Here's the drawing with two shaded views (mm, measured from the low corner). I have some questions. A direction names the side the tool comes from. Give positions to 0.01 mm unless a question says otherwise; leave off trailing zeros. Order: outer loops, then holes, each group sorted by start corner. A loop starts at its lowest first (then second) coordinate and runs counter-clockwise, first axis right, second up. Notation, with made-up numbers: M -21.75,50.25 L 30.25,50.25 A27 ccw 30.25,80.25 Z; hole C 63.25,-13.75 d11. An arc over 180 degrees is marked long. Write each question's results on one line, items separated by ' | '.
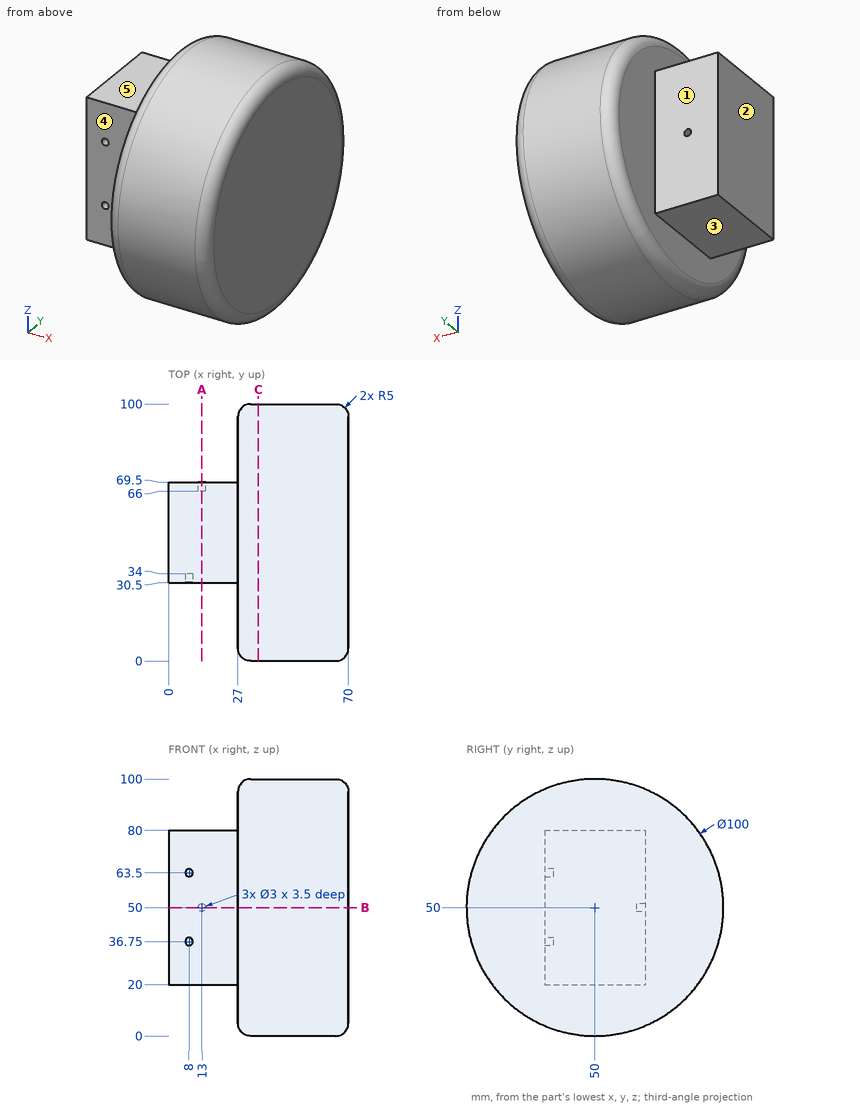
(1) For the marked faces 1, 2, 3, 4 and 5, which set-ups out of +Z, -Z, +X, -X, +Y, -Y let a thin tool reach every point of the face, with its end or its side?
Data:
face 1: +Z, -Z, -X, +Y | face 2: +Z, -Z, -X, +Y, -Y | face 3: -Z, -X, +Y, -Y | face 4: +Z, -Z, -X, -Y | face 5: +Z, -X, +Y, -Y
(2) I need wall thicknesses on L1, parallel to X at y = 68, z = 50; L2, parallel to Z at x = 6.5, y = 57.5; L3, parallel to Y at x = 5, z = 35.5. Which ranges of each line are inside material? Lowest first, please. Write a range as from..to.
Data:
L1: x = 0..11.5, 14.5..70 | L2: z = 20..80 | L3: y = 30.5..69.5
(3) Imagine slicing it at B-B, the plane z = 50. Write out the boundary of the cut face in (x, y).
Data:
outline: M 0,30.5 L 27,30.5 L 27,5 A5 ccw 32,0 L 65,0 A5 ccw 70,5 L 70,95 A5 ccw 65,100 L 32,100 A5 ccw 27,95 L 27,69.5 L 14.5,69.5 L 14.5,66 L 11.5,66 L 11.5,69.5 L 0,69.5 Z
(4) Imagine slicing it at A-A, the plane x = 13. Write out the boundary of the cut face in (y, z).
Data:
outline: M 30.5,20 L 69.5,20 L 69.5,48.5 L 66,48.5 L 66,51.5 L 69.5,51.5 L 69.5,80 L 30.5,80 Z
(5) Will these pins go through, and if not, where does the flat tip stop? P1, Ø21.5, axis at x = 18, z = 42, coming from the +Y side; P2, Ø3, axis at x = 17, z = 76, coming from the +Y side; P3, Ø4, axis at x = 13, z = 50, coming from the -Y side.
Data:
P1: stops at y = 98.27 | P2: stops at y = 69.5 | P3: stops at y = 30.5
(6) Imagine slicing it at C-C, the plane x = 35. Write out the boundary of the cut face in (y, z).
Data:
outline: C 50,50 d100
